CAD build for the part. Positions are in the model's coordinates, mm. Face numbers are marked on the shaded views. A direction names the side the tool comes from. Give positions to 0.01 mm unless a question says otherwise; leave off trailing zeros. Loops run counter-clockwise (first coordinate to the right, second up) from the corner with the lowest first, then second, coordinate; pieces in that order, holes last.
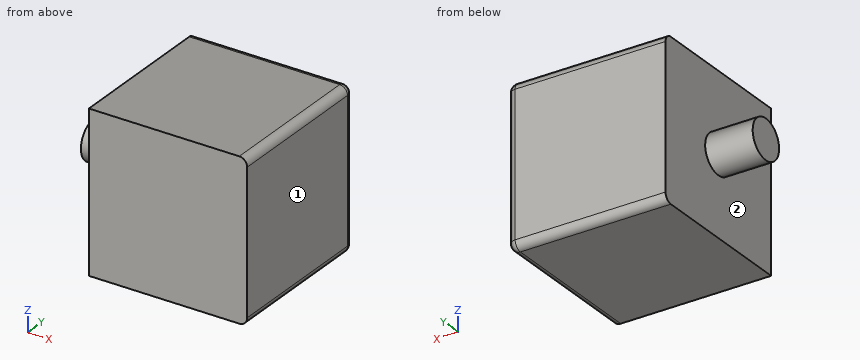
```python
from build123d import *

# Parameters (mm, degrees)
SKETCH1_W           = 20
SKETCH1_H           = 20
BOSS_EXTRUDE1_DEPTH = 20
SKETCH2_R           = 2.5
BOSS_EXTRUDE2_DEPTH = 6
FILLET1_R           = 1


with BuildPart() as part:
    # Sketch1 → Boss-Extrude1 (new body)
    with BuildSketch(Plane(origin=(0, 0, 0), x_dir=(1, 0, 0), z_dir=(0, 1, 0))):
        Rectangle(SKETCH1_W, SKETCH1_H)
    extrude(amount=BOSS_EXTRUDE1_DEPTH)

    # Sketch2 → Boss-Extrude2 (add)
    with BuildSketch(Plane.ZY.offset(10)):
        with Locations((0, 10)):
            Circle(SKETCH2_R)
    extrude(amount=BOSS_EXTRUDE2_DEPTH)

    # Fillet1
    fillet1_edges = [part.edges().sort_by_distance(p)[0] for p in [
        (10, 20, 0),
        (0, 20, -10),
        (10, 10, -10),
        (10, 10, 10),
        (0, 20, 10),
    ]]
    fillet(fillet1_edges, radius=FILLET1_R)


solid = part.part
```
1. Saw through at D-D, the plane y = 1. List the corners of the cut face in (x, z), and give its area (3 significant figures).
Responses:
outline: (-10, -10) - (9, -10) arc R1 ccw to (10, -9) - (10, 9) arc R1 ccw to (9, 10) - (-10, 10) - close
area: 400 mm2
2. Saw through at C-C, the plane z = -5. List the corners of the cut face in (x, y), and give its area (3 significant figures).
Responses:
outline: (-10, 0) - (10, 0) - (10, 19) arc R1 ccw to (9, 20) - (-10, 20) - close
area: 400 mm2
3. Saw through at A-A, the plane z = 0. List the corners of the cut face in (x, y).
Responses:
outline: (-16, 7.5) - (-10, 7.5) - (-10, 0) - (10, 0) - (10, 19) arc R1 ccw to (9, 20) - (-10, 20) - (-10, 12.5) - (-16, 12.5) - close
4. Saw through at B-B, the plane y = 10. List the corners of the cut face in (x, z).
Responses:
outline: (-16, -2.5) - (-10, -2.5) - (-10, -10) - (9, -10) arc R1 ccw to (10, -9) - (10, 9) arc R1 ccw to (9, 10) - (-10, 10) - (-10, 2.5) - (-16, 2.5) - close
5. Drop flat-ended pins along their axis: pin 1 (5 mm diameter, centred on x = 1.5, z = -7.5, fed in from -Y); pin 2 (6 mm diameter, centred on y = 11, z = -7.5, fed in from -X). Give the stop position or say it passes through.
Responses:
pin 1: stops at y = 0
pin 2: stops at x = -10
6. Probe line 1 along X through (y, z) = (18, 0.5); line 2 along Y through (x, z) = (-11.5, -1); line 3 along Y through (x, z) = (-12.75, -1.75). List the from-to ranges inside material, lowest first.
Responses:
line 1: x = -10 to 10
line 2: y = 7.71 to 12.29
line 3: y = 8.21 to 11.79
7. Tool access for the marked faces 1 and 2: list every direction of +Z, -Z, +X, -X, +Y, -Y with a clear straight run to the whole face (end or side of a thin tool).
Responses:
face 1: +Z, -Z, +X, +Y, -Y
face 2: -X
